from build123d import *

# Parameters (mm, degrees)
F0_W           = 101.6
F0_H           = 50.8
F1_DEPTH       = 12.7
F3_D           = 3.175
F3_CBORE_D     = 6.35
F3_CBORE_DEPTH = 6.35
F5_DEPTH       = 101.601
F6_D           = 3.175
F6_CBORE_D     = 6.35
F6_CBORE_DEPTH = 6.35
F7_D           = 3.175
F7_CBORE_D     = 6.35
F7_CBORE_DEPTH = 6.35
F8_D           = 3.175
F8_CBORE_D     = 6.35
F8_CBORE_DEPTH = 6.35


with BuildPart() as f1:
    # F0 (on Front) → F1 (new body)
    with BuildSketch(Plane.XZ):
        with Locations((50.8, 25.4)):
            Rectangle(F0_W, F0_H)
    extrude(amount=F1_DEPTH)

    # F3 (through all)
    with Locations(Plane.XZ.offset(12.7)):
        with Locations((6.35, 7.101479)):
            CounterBoreHole(F3_D / 2, F3_CBORE_D / 2, F3_CBORE_DEPTH)

    # F4 (on face) → F5 (cut, through all)
    with BuildSketch(Plane(origin=(0, 0, 0), x_dir=(0, -1, 0), z_dir=(-1, 0, 0))):
        Polygon((12.7, 33.6042), (8.2042, 38.1), (8.2042, 12.7), (12.7, 17.1958), align=None)
    extrude(amount=-F5_DEPTH, mode=Mode.SUBTRACT)

    # F6 (through all)
    with Locations(Plane.XZ.offset(12.7)):
        with Locations((6.35, 43.698521)):
            CounterBoreHole(F6_D / 2, F6_CBORE_D / 2, F6_CBORE_DEPTH)

    # F7 (through all)
    with Locations(Plane.XZ.offset(12.7)):
        with Locations((95.25, 43.698521)):
            CounterBoreHole(F7_D / 2, F7_CBORE_D / 2, F7_CBORE_DEPTH)

    # F8 (through all)
    with Locations(Plane.XZ.offset(12.7)):
        with Locations((95.25, 7.101479)):
            CounterBoreHole(F8_D / 2, F8_CBORE_D / 2, F8_CBORE_DEPTH)


solid = f1.part
Check sheet for the modelled part. Datum: model origin and axes. Units: mm. A direction names the side the tool comes from. Give positions to 0.01 mm unless a question says otherwise; leave off trailing zeros. Loops run counter-clockwise (first coordinate to the right, second up) from the corner with the lowest first, then second, coordinate; pieces in that order, holes last. Notation, with made-up numbers: M -5,-27.5 L 34,-27.5 A28 ccw 34,-4.5 Z; hole C 29.5,-7 d5. An arc over 180 degrees is marked long. Use a Markdown table: item, result. Add a question column.
Q1. Sectioned sample at A-A, the plane x = 6.35. Record the cut outline in (y, z), then the cut area to 3 significant figures.
Q2. Sectioned sample at C-C, the plane x = 77.5. Record the cut outline in (y, z), then the cut area to 3 significant figures.
Q3. Scan lines: line 1 along X through (y, z) = (-5.5, 7); line 2 along Z through (x, y) = (6.35, -3.75); line 3 along Z through (x, y) = (5, -10). Record each from-to range of solid material in increasing order. Write a range as [from, to].
Q4. Mould release check, pull along Z, two halves, no side actions. Record for faces 4 (the flat face through (50, -6, 0)), 5 (the flat face through (8, -6.35, 42)), 6 (the flat face through (50, 0, 26)): pulls with the +Z half, pulls with the -Z half, needs draft (parallel to the pull), parting line crosses it, or undercut.
Q5. Go/stop test with a flat-tipped pin: pin 1 (4 mm diameter, centred on x = 95.25, z = 43.7, fed in from -Y). Record where the tip stops, or that it passes through.
Q6. Sectioned sample at D-D, the plane z = 31. Record the cut outline in (x, y).
Q7. Sectioned sample at B-B, the plane z = 36.5. Record the cut outline in (x, y).
Q8. Tool access check on faces 1 (the flat face through (0, -6, 25)), 2 (the flat face through (50, -8.204, 26)), 3 (the flat face through (96, -6.35, 9)). Record the directions out of +Z, -Z, +X, -X, +Y, -Y that give a thin tool (end or side, any length) a straight path to the whole face; none if there is none.
Verdict:
| question | item | result |
|---|---|---|
| 1 | outline | M -12.7,0 L 0,0 L 0,5.51 L -6.35,5.51 L -6.35,3.93 L -12.7,3.93 Z; M -12.7,10.28 L -6.35,10.28 L -6.35,8.69 L 0,8.69 L 0,42.11 L -6.35,42.11 L -6.35,40.52 L -12.7,40.52 L -12.7,33.6 L -8.2,38.1 L -8.2,12.7 L -12.7,17.2 Z; M -12.7,46.87 L -6.35,46.87 L -6.35,45.29 L 0,45.29 L 0,50.8 L -12.7,50.8 Z |
| 1 | area | 430 mm^2 |
| 2 | outline | M -12.7,0 L 0,0 L 0,50.8 L -12.7,50.8 L -12.7,33.6 L -8.2,38.1 L -8.2,12.7 L -12.7,17.2 Z |
| 2 | area | 551 mm^2 |
| 3 | line 1 | [0, 4.77], [7.93, 93.67], [96.83, 101.6] |
| 3 | line 2 | [0, 5.51], [8.69, 42.11], [45.29, 50.8] |
| 3 | line 3 | [0, 4.23], [9.98, 14.5], [36.3, 40.82], [46.57, 50.8] |
| 4 | face 4 | pulls with the -Z half |
| 4 | face 5 | undercut |
| 4 | face 6 | needs draft |
| 5 | pin 1 | y = -6.35 |
| 6 | outline | M 0,-8.2 L 101.6,-8.2 L 101.6,0 L 0,0 Z |
| 7 | outline | M 0,-12.7 L 101.6,-12.7 L 101.6,-9.8 L 0,-9.8 Z; M 0,-8.2 L 101.6,-8.2 L 101.6,0 L 0,0 Z |
| 8 | face 1 | +Z, -Z, -X, +Y, -Y |
| 8 | face 2 | +X, -X |
| 8 | face 3 | -Y |
